The listing builds one solid part. Answer for the finished solid, in the listing's coordinates (mm). Face numbers are marked on the shaded views. A direction names the side the tool comes from. Coordinates: 2 decimals unless noted, no trailing zeros. Order: outer loops, then holes, each group sorted by start corner. A loop starts at its lowest first (then second) coordinate and runs counter-clockwise, first axis right, second up. Notation, with made-up numbers: (33, -32.75) -> (58, -32.75) arc R23 cw to (58, 5.25) -> close; hole circle Ø6 at (17, 48). An arc over 180 degrees is marked (long way). Return JSON: item names as keys, results as strings.
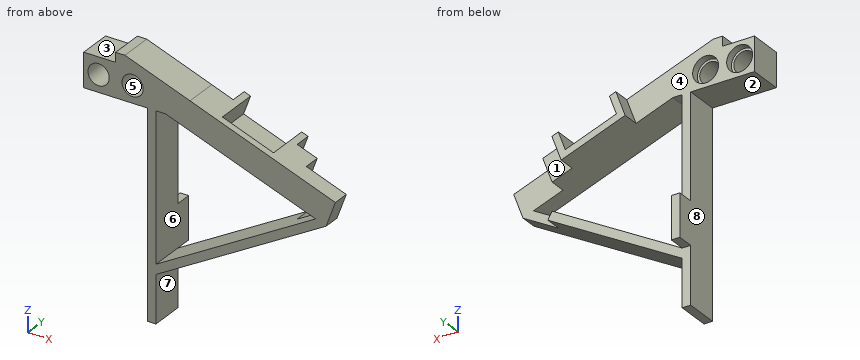
Autodesk Inventor part; units mm, degrees
ref_plane "YZ Plane" through (0, 0, 0) normal (1, 0, 0) x (0, 1, 0)
ref_plane "XZ Plane" through (0, 0, 0) normal (0, 1, 0) x (-1, 0, 0)
ref_plane "XY Plane" through (0, 0, 0) normal (0, 0, 1) x (1, 0, 0)
sketch "Sketch2" plane through (0, 0, 0) normal (0, 1, 0) x (-1, 0, 0)
  line L0 (7.5, -4) -> (-7.5, -4)
  line L1 (-7.5, -4) -> (-7.5, 4)
  line L2 (-7.5, 4) -> (7.5, 4)
  line L3 (7.5, 4) -> (7.5, -4)
  circle A0 centre (4, 0) radius 2.5
  circle A1 centre (-4, 0) radius 2.5
  line L4 (0, -4) -> (0, 11) construction
  circle A2 centre (0, 11) radius 3.7 construction
  line L5 (-30.3941, -4) -> (1.2655, 7.5231) construction
  line L6 (-17.5, -4) -> (-17.5, 0.6931)
  line L7 (-17.5, 0.6931) -> (0, 7.0625)
  line L8 (0, 7.0625) -> (0, 4)
  line L9 (-17.5, -4) -> (-7.5, -4)
  line L10 (-11.8902, 2.7349) -> (-12.4882, 4.3778) construction
  line L11 (-17.5, 0.6931) -> (-51.6831, -11.7486)
  line L12 (-51.6831, -11.7486) -> (-49.4993, -17.7486)
  circle A3 centre (0, 7.0625) radius 55 construction
  line L13 (0, 14.7) -> (0, 62.0625) construction
  line L14 (-49.4993, -17.7486) -> (-11.7254, -4)
  line L15 (-7.5, -4) -> (-7.5, -41.9969)
  line L16 (-7.5, -41.9969) -> (-49.4993, -17.7486)
  line L17 (-9.5, -4) -> (-9.5, -38.5328)
  line L18 (-9.5, -38.5328) -> (-47.0459, -16.8556)
  line L19 (0, 6.2625) -> (-2.198, 6.2625)
  line L20 (-22.5526, -1.1459) -> (-20.3688, -7.1459)
  line L21 (-20.3688, -7.1459) -> (-35.4039, -12.6183)
  line L22 (-35.4039, -12.6183) -> (-37.5877, -6.6183)
  line L23 (-37.5877, -6.6183) -> (-22.5526, -1.1459)
  line L24 (-9.5, -38.5328) -> (-9.5, -51.9969)
  line L25 (-9.5, -51.9969) -> (-7.5, -51.9969)
  line L26 (-7.5, -51.9969) -> (-7.5, -41.9969)
  arc A4 (0, 47.0625) -> (-37.5877, -6.6183) centre (0, 7.0625) ccw construction
  line L27 (-7.5, -38.5328) -> (-9.5, -38.5328)
  line L28 (-9.5, -38.5328) -> (-9.5, -28.5328)
  line L29 (-9.5, -28.5328) -> (-7.5, -28.5328)
  line L30 (-7.5, -28.5328) -> (-7.5, -38.5328)
  circle A5 centre (4, 0) radius 3.05
  circle A6 centre (-4, 0) radius 3.05
  line L31 (-42.2862, -8.3284) -> (-40.1023, -14.3284)
  line L32 (-40.1023, -20.8645) -> (-41.1023, -22.5965)
  point P0 (0, 0)
  point P1 (7.5, 0)
  point P2 (0, 3.5)
  point P3 (-9.5, -40.8422)
  dimension "d6" = 5
  dimension "d7" = 8
  dimension "d9" = 11
  dimension "d10" = 7.4
  dimension "d11" = 8
  dimension "d12" = 15
  dimension "d13" = 70
  dimension "d14" = 10
  dimension "d21" = 14
  dimension "d25" = 55
  dimension "d27" = 6
  dimension "d35" = 60
  dimension "d36" = 3.5
  dimension "d37" = 2
  dimension "d38" = 2
  dimension "d39" = 0.8
  dimension "d40" = 10
  dimension "d41" = 40
  dimension "d42" = 16
  dimension "d43" = 10
  dimension "d46" = 6.1
  dimension "d47" = 6.1
  dimension "d50" = 10
extrude "Extrusion1" add sketch "Sketch2" along normal blind 7.8 contours L0 L1 L2 L3 | L9 L6 L7 L19 L8 L2 L1 | L15 L29 L17 L9 | L14 L20 L11 L6 L9 | L15 L16 L24 L27 | L24 L16 L32 L18 | L26 L25 L24 L16 | L14 L31 L11 L22
extrude "Wyciągnięcie proste3" add sketch "Sketch2" along normal blind 11.7 contours L15 L27 L17 L29 | L14 L22 L11 L20
extrude "Wyciągnięcie proste4" add sketch "Sketch2" along normal blind 6.1 contours A5 | A6
extrude "Wyciągnięcie proste5" add sketch "Sketch2" along normal blind 3.9 contours L32 L16 L14 L18 | L14 L12 L11 L31
sketch "Szkic6" plane through (2.198, 0, 6.2625) normal (0.342, 0, 0.9397) x (0.9397, 0, -0.342)
  line L0 (21.661, 11.7) -> (37.661, 11.7)
  line L1 (23.261, 11.7) -> (36.061, 11.7)
  line L2 (36.061, 11.7) -> (36.061, 1.6)
  line L3 (36.061, 1.6) -> (23.261, 1.6)
  line L4 (23.261, 1.6) -> (23.261, 11.7)
  line L5 (37.661, 7.8) -> (37.661, 11.7)
  line L6 (21.661, 7.8) -> (21.661, 11.7)
  line L7 (0, 0) -> (52.661, 0)
  point P0 (0.0765, 0)
  point P1 (37.661, 9.75)
  point P2 (21.661, 9.75)
  dimension "d59" = 1.6
  dimension "d60" = 1.6
  dimension "d61" = 1.6
extrude "Wyciągnięcie proste7" cut sketch "Szkic6" against normal blind 4.785
mirror "Odbij1" [suppressed]
equation "\"d38\" = d37"
equation "\"d47\" = d46"
properties part number "blokerv9"
Item 1: The part is cut by section D-D on z = 0. Determine the outline of the cut face in (x, y), plus the area to 3 significant figures.
Answer list:
{"outline": "(-7.5, 0) -> (-6.5, 0) -> (-6.5, 6.1) -> (-7.05, 6.1) -> (-7.05, 7.8) -> (-7.5, 7.8) -> close; (-1.5, 0) -> (1.5, 0) -> (1.5, 6.1) -> (0.95, 6.1) -> (0.95, 7.8) -> (-0.95, 7.8) -> (-0.95, 6.1) -> (-1.5, 6.1) -> close; (6.5, 0) -> (19.4, 0) -> (19.4, 7.8) -> (7.05, 7.8) -> (7.05, 6.1) -> (6.5, 6.1) -> close", "area": "128 mm2"}
Item 2: The part is cut by section A-A on x = -4. Determine the outline of the cut face in (y, z).
Answer list:
{"outline": "(0, -4) -> (7.8, -4) -> (7.8, -3.05) -> (6.1, -3.05) -> (6.1, -2.5) -> (0, -2.5) -> close; (0, 2.5) -> (6.1, 2.5) -> (6.1, 3.05) -> (7.8, 3.05) -> (7.8, 4) -> (0, 4) -> close"}
Item 3: Determine the mould class of the marked faces 5, 6, 7 and 8 for opening direction X: pulls with the +X half, pulls with the -X half, needs draft (parallel to the pull), parting line crosses it, or undercut.
Answer list:
{"face 5": "undercut", "face 6": "undercut", "face 7": "pulls with the +X half", "face 8": "pulls with the -X half"}
Item 4: The part is cut by section C-C on y = 9.5. Determine the outline of the cut face in (x, z), plus the area to 3 significant figures.
Answer list:
{"outline": "(7.5, -38.53) -> (9.5, -38.53) -> (9.5, -28.53) -> (7.5, -28.53) -> close; (20.37, -7.15) -> (35.4, -12.62) -> (37.59, -6.62) -> (36.08, -6.07) -> (34.45, -10.57) -> (22.42, -6.19) -> (24.06, -1.69) -> (22.55, -1.15) -> close", "area": "60.9 mm2"}
Item 5: Flat-ended cylindrical pins translate along their axes: pin 1 (3 mm diameter, centred on x = 4, z = 0, fed in from +Y); pin 2 (2 mm diameter, centred on x = 38, z = -11.5, fed in from +Y); pin 3 (0.7 mm diameter, centred on x = 11, y = 5.5, fed in from -Z); pin 4 (6 mm diameter, centred on y = 8, z = -40.5, fed in from +X). Find the tip coordinate at first contact, or state that the pin passes through.
Answer list:
{"pin 1": "through", "pin 2": "y = 7.8", "pin 3": "z = -40.18", "pin 4": "x = 15.28"}
Item 6: Find the intervals of material crossed by probe 1 along Z at (x, y) = (-4, 7.15); probe 2 along Z at (x, y) = (-4, 2.5); probe 3 along X at (y, z) = (8.75, -38), in increasing order.
Answer list:
{"probe 1": "-4 to -3.05, 3.05 to 4", "probe 2": "-4 to -2.5, 2.5 to 4", "probe 3": "7.5 to 9.5"}
Item 7: The part is cut by section B-B on z = -25. Determine the outline of the cut face in (x, y), plus the area to 3 significant figures.
Answer list:
{"outline": "(7.5, 0) -> (9.5, 0) -> (9.5, 7.8) -> (7.5, 7.8) -> close; (32.94, 0) -> (36.94, 0) -> (36.94, 7.8) -> (32.94, 7.8) -> close", "area": "46.8 mm2"}
Item 8: Which of the six approach directions +Z, -Z, +X, -X, +Y, -Y give full straight-line access (tool end or side, diameter ignored) to the marked faces 1, 2, 3 and 4?
Answer list:
{"face 1": "-Z, +X, +Y", "face 2": "-Z, -X, +Y, -Y", "face 3": "+Z, -X, +Y, -Y", "face 4": "+Z, -X, +Y"}
